Print and shaded views of the part. All mm, measured from the part's lowest x, y and z. Round coordinates to 2 decimals unless told otherwise and drop trailing zeros. Loops run counter-clockwise (first coordinate to the right, second up) from the corner with the lowest first, then second, coordinate; pieces in that order, holes last. Notation, with made-up numbers: (82, 30.5) -> (100, 30.5) arc R19 ccw to (100, 49.5) -> close; hole circle Ø10 at (-39.75, -29.5). An arc over 180 degrees is marked (long way). Answer as CSV lines item,"result".
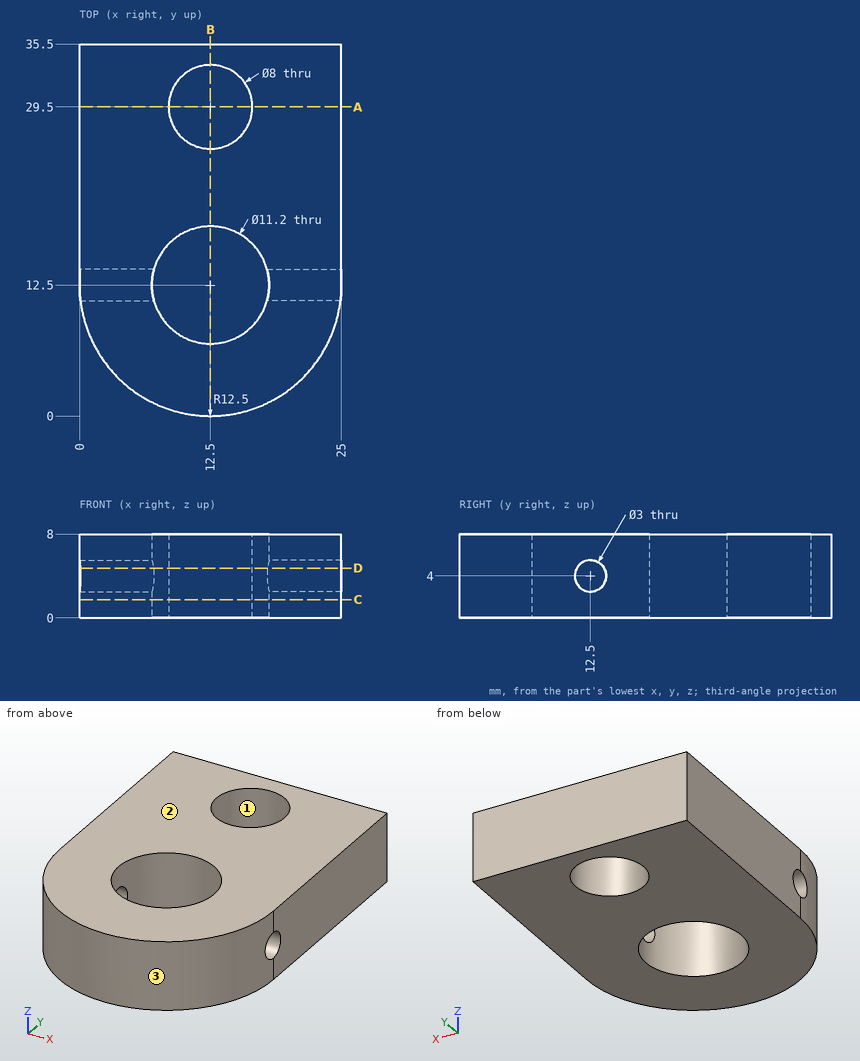
Q1. Two-plate mould, pull along X, no slides. Class the marked faces 1, 2 and 3: pulls with the +X half, pulls with the -X half, needs draft (parallel to the pull), parting line crosses it, or undercut.
Geometry results:
face 1,"undercut"
face 2,"needs draft"
face 3,"parting line crosses it"
Q2. Drill centre lines: line 1 along Y through (x, z) = (12.25, 1.25); line 2 along Y through (x, z) = (11.25, 0.5); line 3 along X through (y, z) = (9.5, 6). Where is each one in solid material? Low to high.
Geometry results:
line 1,"0 to 6.91, 18.09 to 25.51, 33.49 to 35.5"
line 2,"0.06 to 7.04, 17.96 to 25.7, 33.3 to 35.5"
line 3,"0.37 to 7.77, 17.23 to 24.63"
Q3. Saw through at B-B, the plane x = 12.5. Write the cut outline in (y, z), then the cut area to 3 significant figures.
Geometry results:
outline,"(0, 0) -> (6.9, 0) -> (6.9, 8) -> (0, 8) -> close; (18.1, 0) -> (25.5, 0) -> (25.5, 8) -> (18.1, 8) -> close; (33.5, 0) -> (35.5, 0) -> (35.5, 8) -> (33.5, 8) -> close"
area,"130 mm2"
Q4. Saw through at C-C, the plane z = 1.75. Write the cut outline in (x, y), then the cut area to 3 significant figures.
Geometry results:
outline,"(0, 12.5) arc R12.5 ccw to (25, 12.5) -> (25, 35.5) -> (0, 35.5) -> close; hole circle Ø11.2 at (12.5, 12.5); hole circle Ø8 at (12.5, 29.5)"
area,"672 mm2"
Q5. Saw through at A-A, the plane y = 29.5. Write the cut outline in (x, z).
Geometry results:
outline,"(0, 0) -> (8.5, 0) -> (8.5, 8) -> (0, 8) -> close; (16.5, 0) -> (25, 0) -> (25, 8) -> (16.5, 8) -> close"
Q6. Saw through at D-D, the plane z = 4.75. Write the cut outline in (x, y), then the cut area to 3 significant figures.
Geometry results:
outline,"(0, 13.8) -> (7.05, 13.8) arc R5.6 cw to (17.95, 13.8) -> (25, 13.8) -> (25, 35.5) -> (0, 35.5) -> close; (0.07, 11.2) arc R12.5 ccw to (24.93, 11.2) -> (17.95, 11.2) arc R5.6 cw to (7.05, 11.2) -> close; hole circle Ø8 at (12.5, 29.5)"
area,"636 mm2"
